```python
from build123d import *

# Parameters (mm, degrees)
SKETCH001_W            = 1.95
SKETCH001_H            = 4.49
PAD_DEPTH              = 0.5
LINEARPATTERN_COUNT    = 2
LINEARPATTERN_PITCH    = 2.54
PAD001_DEPTH           = 0.975
PAD002_DEPTH           = 0.975
PAD003_DEPTH           = 1.58
SKETCH005_W            = 1.95
SKETCH005_H            = 4.5
SKETCH005_H_2          = 4.05
POCKET_DEPTH           = 1
SKETCH006_R            = 0.6
PAD004_DEPTH           = 4.64
LINEARPATTERN001_COUNT = 2
LINEARPATTERN001_PITCH = 6.6
CHAMFER_1_ANGLE        = 20
CHAMFER_1_SIZE         = 0.8
CHAMFER_2_ANGLE        = 20
CHAMFER_2_SIZE         = 0.8


with BuildPart() as part:
    # Sketch001 → Pad (new body)
    with BuildSketch(Plane.YZ):
        with Locations((0, 1.27)):
            Rectangle(SKETCH001_W, SKETCH001_H)
    extrude(amount=-PAD_DEPTH)

    # Sketch → Revolution (revolve)
    with BuildSketch(Plane.XZ):
        with BuildLine():
            Line((0, 0), (0, 0.975))
            Line((0, 0.975), (2.5, 0.975))
            Line((2.5, 0.975), (2.5, 0.775))
            ThreePointArc((2.8, 0), (2.722383, 0.415519), (2.5, 0.775))
            Line((2.8, 0), (0, 0))
        make_face()
    revolution = revolve(axis=Axis((0, 0, 0), (1, 0, 0)))

    # LinearPattern: Revolution ×2
    with Locations(*[(0, 0, i * LINEARPATTERN_PITCH) for i in range(1, LINEARPATTERN_COUNT)]):
        add(revolution)

    # Sketch002 → Pad001 (join, symmetric)
    with BuildSketch(Plane.XZ):
        with BuildLine():
            Line((-0.5, 3.515), (-4.485, 3.515))
            ThreePointArc((-4.485, 3.515), (-6.97048, 2.48548), (-8, 0))
            Line((-8, 0), (-6.05, 0))
            ThreePointArc((-4.485, 1.565), (-5.591622, 1.106622), (-6.05, 0))
            Line((-4.485, 1.565), (-0.5, 1.565))
            Line((-0.5, 1.565), (-0.5, 3.515))
        make_face()
    extrude(amount=PAD001_DEPTH, both=True)

    # Sketch003 → Pad002 (join, symmetric)
    with BuildSketch(Plane.XZ):
        Polygon((-0.5, 0.975), (-3.55, 0.975), (-5.5, -0.975), (-0.5, -0.975), align=None)
    extrude(amount=PAD002_DEPTH, both=True)

    # Sketch004 → Pad003 (join, symmetric)
    with BuildSketch(Plane.XZ):
        Polygon((0, -2.54), (-9.05, -2.54), (-9.05, 0.5), (-3.05, 0.5), (-3.05, -1.14), (0, -1.14), align=None)
    extrude(amount=PAD003_DEPTH, both=True)

    # Sketch005 (on Face27 of Pad003) → Pocket (cut)
    with BuildSketch(Plane.YX.offset(2.54)):
        with Locations((0, -2.25)):
            Rectangle(SKETCH005_W, SKETCH005_H)
        with Locations((0, -7.025)):
            Rectangle(SKETCH005_W, SKETCH005_H_2)
    extrude(amount=-POCKET_DEPTH, mode=Mode.SUBTRACT)

    # Sketch006 → Pad004 (join)
    with BuildSketch(Plane.XY):
        with Locations((-1.4, 0)):
            Circle(SKETCH006_R)
    pad004 = extrude(amount=-PAD004_DEPTH)

    # LinearPattern001: Pad004 ×2
    with Locations(*[(-i * LINEARPATTERN001_PITCH, 0, 0) for i in range(1, LINEARPATTERN001_COUNT)]):
        add(pad004)

    # Chamfer 1
    chamfer_1_edges = [part.edges().sort_by_distance(p)[0] for p in [
        (-2, 0, -4.64),
    ]]
    chamfer_1_side = part.faces().sort_by_distance((-2, 0, -3.09))[0]
    chamfer(chamfer_1_edges, length=CHAMFER_1_SIZE, angle=CHAMFER_1_ANGLE, reference=chamfer_1_side)

    # Chamfer 2
    chamfer_2_edges = [part.edges().sort_by_distance(p)[0] for p in [
        (-8.6, 0, -4.64),
    ]]
    chamfer_2_side = part.faces().sort_by_distance((-8.6, 0, -3.09))[0]
    chamfer(chamfer_2_edges, length=CHAMFER_2_SIZE, angle=CHAMFER_2_ANGLE, reference=chamfer_2_side)


solid = part.part
```
Part model, mm, in its own coordinate system. A direction names the side the tool comes from. Round coordinates to 2 decimals unless told otherwise and drop trailing zeros. Write each loop counter-clockwise with the first axis right and the second up, starting at its lowest first coordinate (ties: lowest second). Pieces come first, ordered by that corner, then holes.
Item 1: Cut at A-A, the plane x = -3.75. Give the cut face in (y, z) (3 decimals), plus the area to 3 significant figures.
Results:
outline: (-1.58, -2.54) - (-0.975, -2.54) - (-0.975, -1.54) - (0.975, -1.54) - (0.975, -2.54) - (1.58, -2.54) - (1.58, 0.5) - (0.975, 0.5) - (0.975, 0.775) - (-0.975, 0.775) - (-0.975, 0.5) - (-1.58, 0.5) - close; (-0.975, 1.565) - (0.975, 1.565) - (0.975, 3.515) - (-0.975, 3.515) - close
area: 12.0 mm2
Item 2: Two-plate mould, pull along Z, no slides. Class faces 1 (the flat face through (-3, 0.975, 2)), 2 (the flat face through (-3, 0, 1.565)), 3 (the flat face through (-7, 0, -1.54)): +Z half, -Z half, draft (parallel to the pull), parting line (faces both ways), or undercut.
Results:
face 1: draft
face 2: undercut
face 3: -Z half
Item 3: Cut at B-B, the plane x = -1.4. Give the cut face in (y, z) (3 decimals).
Results:
outline: (-1.58, -2.54) - (-0.975, -2.54) - (-0.975, -1.54) - (-0.6, -1.54) - (-0.6, -3.84) - (-0.309, -4.64) - (0.309, -4.64) - (0.6, -3.84) - (0.6, -1.54) - (0.975, -1.54) - (0.975, -2.54) - (1.58, -2.54) - (1.58, -1.14) - (0.6, -1.14) - (0.6, -0.975) - (0.975, -0.975) - (0.975, 0.975) - (-0.975, 0.975) - (-0.975, -0.975) - (-0.6, -0.975) - (-0.6, -1.14) - (-1.58, -1.14) - close; (-0.975, 1.565) - (0.975, 1.565) - (0.975, 3.515) - (-0.975, 3.515) - close
Item 4: Probe L1, parallel to Z at x = -3.25, y = -0.15 (3 decimals); L2, parallel to Y at x = -1, z = -2.5 (3 decimals); L3, parallel to X at y = 1.4, z = 0. List the from-to ranges inside material, lowest first.
Results:
L1: z = -1.54 to 0.975, 1.565 to 3.515
L2: y = -1.58 to -0.975, -0.447 to 0.447, 0.975 to 1.58
L3: x = -9.05 to -3.05
Item 5: Drop flat-ended pins along their axis: pin 1 Ø1.5 at (x, y) = (-6, 1) entering from -Z; pin 2 Ø0.6 at (y, z) = (-0.5, 1.5) entering from +X. Give the stop position or say it passes through.
Results:
pin 1: stops at z = -2.54
pin 2: stops at x = 2.5
Item 6: Cut at D-D, the plane z = -4. Give the cut face in (x, y).
Results:
outline: circle Ø1.08 at (-8, 0); circle Ø1.08 at (-1.4, 0)
Item 7: Which spindle directions (+Z, -Z, +X, -X, +Y, -Y) get a long thin tool onto all of the face, cutting with end or side? Do faces 4 (the flat face through (-7, -0.975, -2)), 5 (the flat face through (-2, 0, 0.975)), 6 (the flat face through (-2.2, 0, -0.975)), 7 (the flat face through (-2, 0.975, -2)). Say none if no direction does.
Results:
face 4: -Z, -X
face 5: +Y, -Y
face 6: none
face 7: -Z, +X
Item 8: Cut at C-C, the plane y = -1.2. Give the cut face in (x, z).
Results:
outline: (-9.05, -2.54) - (0, -2.54) - (0, -1.14) - (-3.05, -1.14) - (-3.05, 0.5) - (-9.05, 0.5) - close
